Work out the finished part from the listing and answer in its coordinate system (mm). Face numbers are marked on the shaded views. Round coordinates to 2 decimals unless told otherwise and drop trailing zeros. Write each loop counter-clockwise with the first axis right and the second up, starting at its lowest first coordinate (ties: lowest second). Pieces come first, ordered by that corner, then holes.
from build123d import *


with BuildPart() as part:
    # Sketch1 → Revolve1 (revolve)
    with BuildSketch(Plane.XY, mode=Mode.PRIVATE) as revolve1_sk:
        with BuildLine():
            Line((38.0492, 0), (35.819999251, 0.59731254))
            ThreePointArc((35.819999251, 0.59731254), (33.104565031, 2.411707679), (32.0548, 5.504215738))
            Line((32.0548, 5.504215738), (32.0548, 76.2))
            Line((32.0548, 76.2), (29.5148, 76.2))
            Line((29.5148, 76.2), (29.5148, -2.54))
            Line((29.5148, -2.54), (63.5, -2.54))
            Line((63.5, -2.54), (63.5, 0))
            Line((63.5, 0), (38.0492, 0))
        make_face()
    revolve(revolve1_sk.sketch.rotate(Axis((0, 0, 0), (0, 1, 0)), 90), axis=Axis((0, 0, 0), (0, 1, 0)))


solid = part.part
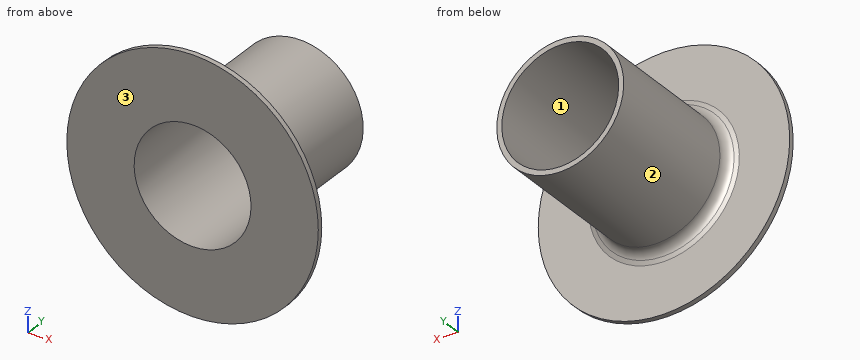
Q1. Find section B-B (z = 0). Determine the outline of the cut face in (x, y).
Q2. Find section C-C (y = 30). Determine the outline of the cut face in (x, z), plus the area to 3 significant figures.
Q3. Given pin 1 (12 mm diameter, centred on x = 26, y = 54, fed in from +Z); pin 2 (3 mm diameter, centred on y = 51.5, z = 5.5, fed in from -X); pin 3 (1.5 mm diameter, centred on x = -36, z = 41.5, fed in from +Y), each flat-ended and moving along its own axis, determine where each tip first touches the part or whether it passes through.
Q4. The mould has two halves that part along Z. Classify the marked faces 1, 2 and 3: +Z half, -Z half, draft (parallel to the pull), parting line (faces both ways), or undercut.
Q5. Find section A-A (x = 0). Determine the outline of the cut face in (y, z).
Q6. Find section D-D (x = 41.5). Determine the outline of the cut face in (y, z), plus the area to 3 significant figures.
Q7. Find the intervals of material crossed by L1, parallel to X at y = 60, z = 0; L2, parallel to Y at x = -44, z = 4; L3, parallel to Z at x = 1, y = 72, in increasing order.
Report:
1. outline: (-63.5, -2.54) - (-29.51, -2.54) - (-29.51, 76.2) - (-32.05, 76.2) - (-32.05, 5.5) arc R5.08 cw to (-35.82, 0.6) - (-38.05, 0) - (-63.5, 0) - close; (29.51, -2.54) - (63.5, -2.54) - (63.5, 0) - (38.05, 0) - (35.82, 0.6) arc R5.08 cw to (32.05, 5.5) - (32.05, 76.2) - (29.51, 76.2) - close
2. outline: circle Ø64.11 at (0, 0); hole circle Ø59.03 at (0, 0)
2. area: 491 mm2
3. pin 1: stops at z = 25.05
3. pin 2: stops at x = -31.8
3. pin 3: stops at y = 0
4. face 1: undercut
4. face 2: parting line
4. face 3: draft
5. outline: (-2.54, -63.5) - (0, -63.5) - (0, -38.05) - (0.6, -35.82) arc R5.08 cw to (5.5, -32.05) - (76.2, -32.05) - (76.2, -29.51) - (-2.54, -29.51) - close; (-2.54, 29.51) - (76.2, 29.51) - (76.2, 32.05) - (5.5, 32.05) arc R5.08 cw to (0.6, 35.82) - (0, 38.05) - (0, 63.5) - (-2.54, 63.5) - close
6. outline: (-2.54, -48.06) - (0, -48.06) - (0, 48.06) - (-2.54, 48.06) - close
6. area: 244 mm2
7. L1: x = -32.05 to -29.51, 29.51 to 32.05
7. L2: y = -2.54 to 0
7. L3: z = -32.04 to -29.5, 29.5 to 32.04
